Here's how the part is built. I have some questions about the finished solid (model axes, mm). A direction names the side the tool comes from. Round coordinates to 2 decimals unless told otherwise and drop trailing zeros. Order: outer loops, then holes, each group sorted by start corner. A loop starts at its lowest first (then second) coordinate and runs counter-clockwise, first axis right, second up. Notation, with made-up numbers: (-35.5, 76.25) -> (21.5, 76.25) arc R16 cw to (21.5, 86.25) -> close; hole circle Ø11 at (43.25, 66.25). An arc over 180 degrees is marked (long way). Use a Markdown table: item, result. Add a question column.
(1) If I drill on probe 1 along Y at (x, z) = (2, 4.25); probe 2 along Z at (x, y) = (0, -3.5); probe 3 along Z at (x, y) = (4, -7.25), over which ranges is the centre line in solid material (lowest first)?
(2) I want a section at D-D, the plane x = -3.25. Please give me the cut outline in (y, z), then the cut area to 3 significant figures.
(3) I'm going to push flat-ended pins straight in: P1, Ø1.5, axis at x = 5, y = 6, coming from the +Z side; P2, Ø5, axis at y = 1, z = 7.5, coming from the -X side; P3, Ø1.5, axis at x = -1, y = -0.5, coming from the +Z side. Where does each tip first touch, or does it pass through?
(4) Thinking about a two-plate mould opening in X: for faces 3 (the face through (-7.99, -0.16, 1.49)), 4 (the face through (0, 0, 6)), 5 (the face through (0, -11.5, 4)), which applies, pulls with the +X half, pulls with the -X half, needs draft (parallel to the pull), parting line crosses it, or undercut?
(5) I want a section at B-B, the plane x = 0. Please give me the cut outline in (y, z), then the cut area to 3 significant figures.
(6) I want a section at A-A, the plane y = 4.5. Please give me the cut outline in (x, z), then the cut area to 3 significant figures.
(7) I want a section at C-C, the plane z = 9. Please give me the cut outline in (x, y).
(8) On a 3-axis mill with a long thin cutter (end or side, diameter ignored), from which of +Z, -Z, +X, -X, +Y, -Y can I reach the whole of each face in a straight line? I mean faces 1 (the face through (5.73, -0.16, 6.86)), 2 (the face through (0, 9.839, 4)). Say none if no direction works.
from build123d import *

# Parameters (mm, degrees)
F2_DEPTH = 11.5
F3_W     = 20
F3_H     = 1.5
F4_DEPTH = 12.5


with BuildPart() as f2:
    # F1 (on Front) → F2 (new body, symmetric)
    with BuildSketch(Plane.XZ):
        with BuildLine():
            ThreePointArc((2.8284271247, 10), (0, 6), (-2.8284271247, 10))
            Line((-2.8284271247, 10), (-3.9100694971, 10))
            Line((-3.9100694971, 10), (-7.5, 3.8031570148))
            ThreePointArc((-7.5, 3.8031570148), (-8.011027857, 1.9015785074), (-7.5, 0))
            Line((-7.5, 0), (7.5, 0))
            ThreePointArc((7.5, 0), (8.011027857, 1.9015785074), (7.5, 3.8031570148))
            Line((7.5, 3.8031570148), (3.9100694971, 10))
            Line((3.9100694971, 10), (2.8284271247, 10))
        make_face()
    extrude(amount=F2_DEPTH, both=True)

    # F3 (on Right) → F4 (cut, symmetric)
    with BuildSketch(Plane.YZ):
        with Locations((-0.1611583866, 3.75)):
            Rectangle(F3_W, F3_H)
    extrude(amount=F4_DEPTH, both=True, mode=Mode.SUBTRACT)


solid = f2.part
Taken from the geometry:
| question | item | result |
|---|---|---|
| 1 | probe 1 | y = -11.5 to -10.16, 9.84 to 11.5 |
| 1 | probe 2 | z = 0 to 3, 4.5 to 6 |
| 1 | probe 3 | z = 0 to 3, 4.5 to 9.84 |
| 2 | outline | (-11.5, 0) -> (11.5, 0) -> (11.5, 10) -> (-11.5, 10) -> close; hole (-10.16, 3) -> (9.84, 3) -> (9.84, 4.5) -> (-10.16, 4.5) -> close |
| 2 | area | 200 mm2 |
| 3 | P1 | stops at z = 9.41 |
| 3 | P2 | stops at x = -6.81 |
| 3 | P3 | stops at z = 6.56 |
| 4 | face 3 | pulls with the -X half |
| 4 | face 4 | undercut |
| 4 | face 5 | needs draft |
| 5 | outline | (-11.5, 0) -> (11.5, 0) -> (11.5, 6) -> (-11.5, 6) -> close; hole (-10.16, 3) -> (9.84, 3) -> (9.84, 4.5) -> (-10.16, 4.5) -> close |
| 5 | area | 108 mm2 |
| 6 | outline | (-7.85, 3) arc R3.79 ccw to (-7.5, 0) -> (7.5, 0) arc R3.79 ccw to (7.85, 3) -> close; (-7.1, 4.5) -> (7.1, 4.5) -> (3.91, 10) -> (2.83, 10) arc R3 cw (long way) to (-2.83, 10) -> (-3.91, 10) -> close |
| 6 | area | 87.8 mm2 |
| 7 | outline | (-4.49, -11.5) -> (-3, -11.5) -> (-3, 11.5) -> (-4.49, 11.5) -> close; (3, -11.5) -> (4.49, -11.5) -> (4.49, 11.5) -> (3, 11.5) -> close |
| 8 | face 1 | +Z, +X, +Y, -Y |
| 8 | face 2 | +X, -X |
